```python
from build123d import *

# Parameters (mm, degrees)
SKETCH_1_R          = 3.2
EXTRUDE_1_DEPTH     = 30
FILLET_1_R          = 4
SKETCH_2_R          = 3.1
CUT_EXTRUDE_1_DEPTH = 47.69047012
SKETCH_3_W          = 22.462925105
SKETCH_3_H          = 21
CUT_EXTRUDE_2_DEPTH = 47.69047012
CHAMFER_1_SIZE      = 2.2
CHAMFER_2_SIZE      = 2.2
CHAMFER_3_SIZE      = 2.2


with BuildPart() as part:
    # Эскиз1 → Бобышка-Вытянуть1 (new body)
    with BuildSketch(Plane(origin=(0, 0, 0), x_dir=(1, 0, 0), z_dir=(0, 1, 0))):
        with BuildLine():
            Line((-32, 8.5), (-1.538396133, 8.5))
            ThreePointArc((-1.538396133, 8.5), (3.466562042, 7.016276971), (6.85424835, 3.044549155))
            ThreePointArc((6.85424835, 3.044549155), (3.352656053, -6.708926694), (-6.549763987, -3.653846154))
            ThreePointArc((-6.549763987, -3.653846154), (-10.952950163, 0.847797982), (-17.029386366, 2.5))
            Line((-17.029386366, 2.5), (-32, 2.5))
            Line((-32, 2.5), (-32, 8.5))
        make_face()
        with Locations(Location((0, 0, 0), (0, 0, 270))):
            Circle(SKETCH_1_R, mode=Mode.SUBTRACT)
    extrude(amount=EXTRUDE_1_DEPTH)

    # Скругление1
    fillet_1_edges = [part.edges().sort_by_distance(p)[0] for p in [
        (-32, 30, -5.5),
        (-32, 0, -5.5),
    ]]
    fillet(fillet_1_edges, radius=FILLET_1_R)

    # Эскиз2 → Вырез-Вытянуть1 (cut, through all)
    with BuildSketch(Plane(origin=(0, 0, -8.5), x_dir=(-1, 0, 0), z_dir=(0, 0, -1))):
        with Locations((21, 23)):
            Circle(SKETCH_2_R)
        with Locations((21, 7)):
            Circle(SKETCH_2_R)
    extrude(amount=-CUT_EXTRUDE_1_DEPTH, mode=Mode.SUBTRACT)

    # Эскиз3 → Вырез-Вытянуть2 (cut, through all)
    with BuildSketch(Plane(origin=(0, 0, -8.5), x_dir=(-1, 0, 0), z_dir=(0, 0, -1))):
        with Locations((-2.231462553, 15)):
            Rectangle(SKETCH_3_W, SKETCH_3_H)
    extrude(amount=-CUT_EXTRUDE_2_DEPTH, mode=Mode.SUBTRACT)

    # Фаска1
    chamfer_1_edges = [part.edges().sort_by_distance(p)[0] for p in [
        (0, 30, -3.2),
    ]]
    chamfer(chamfer_1_edges, length=CHAMFER_1_SIZE)

    # Фаска2
    chamfer_2_edges = [part.edges().sort_by_distance(p)[0] for p in [
        (-17.9, 23, -8.5),
    ]]
    chamfer(chamfer_2_edges, length=CHAMFER_2_SIZE)

    # Фаска3
    chamfer_3_edges = [part.edges().sort_by_distance(p)[0] for p in [
        (-17.9, 7, -8.5),
    ]]
    chamfer(chamfer_3_edges, length=CHAMFER_3_SIZE)


solid = part.part
```
Can you work these out from the model? Positions are in its coordinate system, mm. A direction names the side the tool comes from. Round coordinates to 2 decimals unless told otherwise and drop trailing zeros. Loops run counter-clockwise (first coordinate to the right, second up) from the corner with the lowest first, then second, coordinate; pieces in that order, holes last. Notation, with made-up numbers: M 9.5,70 L 30.5,70 A20 cw 30.5,74 Z; hole C 49.5,54 d5. An arc over 180 degrees is marked long. Answer as a JSON object with one key per item and string values. Group by question number.
Q1. Will these pins go through, and if not, where does the flat tip stop? pin 1 (1 mm diameter, centred on x = -18.5, y = 9.5, fed in from -Z); pin 2 (4 mm diameter, centred on x = 2, z = -2.5, fed in from +Y); pin 3 (8 mm diameter, centred on x = -18.5, z = -1.5, fed in from -Y); pin 4 (4 mm diameter, centred on y = 15.5, z = 0.5, fed in from -X).
Q2. We'd pull the mould along X, two halves only. Please class faces 4 (the conical face through (-2.012, 27.907, -2.624)), 5 (the flat face through (-32, 15, -5)), 6 (the flat face through (-2.5, 4.5, -2.4)): +X half, -X half, draft (parallel to the pull), parting line (faces both ways), or undercut.
Q3. Imagine slicing it at A-A, the plane x = -21. Please give me the cut outline in (y, z), then the cut area to 3 significant figures.
Q4. Please list where these lines run through material, in increasing order: L1, parallel to Y at x = -21, z = -4.8; L2, parallel to Z at x = -25, y = 3.5; L3, parallel to Y at x = 1.5, z = 5.25.
Q5. Imagine slicing it at D-D, the plane y = 17. Please give me the cut outline in (x, z), then the cut area to 3 significant figures.
Q6. Imagine slicing it at B-B, the plane x = 0. Please give me the cut outline in (y, z).
Q7. On a 3-axis mill with a long thin cutter (end or side, diameter ignored), from which of +Z, -Z, +X, -X, +Y, -Y can I reach the whole of each face in a straight line? I mean faces 1 (the flat face through (-24, 15, -2.5)), 2 (the flat face through (-2.5, 25.5, -2.4)), 3 (the cylindrical face through (-30.859, 1.203, -5.542)). Say none if no direction works.
Q8. Imagine slicing it at C-C, the plane z = 0. Please give me the cut outline in (x, y).
Findings:
{
 "1": {"pin 1": "stops at z = -7.24", "pin 2": "stops at y = 29.8", "pin 3": "stops at y = 0", "pin 4": "stops at x = -12.23"},
 "2": {"face 4": "undercut", "face 5": "-X half", "face 6": "draft"},
 "3": {"outline": "M 0,-8.5 L 1.7,-8.5 L 3.9,-6.3 L 3.9,-2.5 L 0,-2.5 Z; M 10.1,-6.3 L 12.3,-8.5 L 17.7,-8.5 L 19.9,-6.3 L 19.9,-2.5 L 10.1,-2.5 Z; M 26.1,-6.3 L 28.3,-8.5 L 30,-8.5 L 30,-2.5 L 26.1,-2.5 Z", "area": "95.9 mm2"},
 "4": {"L1": "y = 0 to 3.9, 10.1 to 19.9, 26.1 to 30", "L2": "z = -8.5 to -2.5", "L3": "y = 0 to 4.5, 25.5 to 30"},
 "5": {"outline": "M -32,-8.5 L -9,-8.5 L -9,0.58 A12 cw -17.03,-2.5 L -32,-2.5 Z", "area": "146 mm2"},
 "6": {"outline": "M 0,-8.37 L 4.5,-8.37 L 4.5,-3.2 L 0,-3.2 Z; M 0,3.2 L 4.5,3.2 L 4.5,7.5 L 0,7.5 Z; M 25.5,-8.37 L 30,-8.37 L 30,-5.4 L 27.8,-3.2 L 25.5,-3.2 Z; M 25.5,3.2 L 27.8,3.2 L 30,5.4 L 30,7.5 L 25.5,7.5 Z"},
 "7": {"face 1": "+Z, -X, +Y, -Y", "face 2": "+Z, -Z, +X", "face 3": "+Z, -Z, -X, -Y"},
 "8": {"outline": "M -9.7,0 L -3.2,0 L -3.2,4.5 L -9,4.5 L -9,25.5 L -3.2,25.5 L -3.2,27.8 L -5.4,30 L -9.7,30 Z; M 3.2,0 L 7.5,0 L 7.5,4.5 L 3.2,4.5 Z; M 3.2,25.5 L 7.5,25.5 L 7.5,30 L 5.4,30 L 3.2,27.8 Z"}
}
